Could you check a few things on this model? Use its own coordinates, in mm. Round coordinates to 2 decimals unless told otherwise and drop trailing zeros. Loops run counter-clockwise (first coordinate to the right, second up) from the corner with the lowest first, then second, coordinate; pieces in that order, holes last. Notation, with made-up numbers: (23, 65) -> (55, 65) arc R29 cw to (55, 87) -> close; hole circle Ø8 at (13, -32). An arc over 180 degrees is marked (long way). One line per item, written item: value.
```python
from build123d import *

# Parameters (mm, degrees)
EXTRUDE_1_DEPTH     = 3
SKETCH_2_R          = 1.6
SKETCH_2_R_2        = 2.85
CUT_EXTRUDE_3_DEPTH = 1.5
SKETCH_3_R          = 7.5
SKETCH_3_R_2        = 15.25
CUT_EXTRUDE_4_DEPTH = 3


with BuildPart() as part:
    # 草图1 → 凸台-拉伸1 (new body)
    with BuildSketch(Plane(origin=(0, 0, 0), x_dir=(1, 0, 0), z_dir=(0, 1, 0))):
        Polygon((5, 48), (71, 48), (71, 5), (75, 5), (75, -5), (71, -5), (71, -48), (5, -48), (5, -51), (-5, -51), (-5, -48), (-71, -48), (-71, -5), (-75, -5), (-75, 5), (-71, 5), (-71, 48), (-5, 48), (-5, 51), (5, 51), align=None)
    extrude(amount=EXTRUDE_1_DEPTH)

    # 草图2 → 切除-拉伸3 (cut)
    with BuildSketch(Plane(origin=(0, 3, 0), x_dir=(1, 0, 0), z_dir=(0, 1, 0))):
        with Locations(Location((-61, -33, 0), (0, 0, 270))):
            Circle(SKETCH_2_R)
        with Locations(Location((24, -33, 0), (0, 0, 270))):
            Circle(SKETCH_2_R)
        with Locations(Location((-61, -11, 0), (0, 0, 270))):
            Circle(SKETCH_2_R_2)
        with Locations(Location((24, -11, 0), (0, 0, 270))):
            Circle(SKETCH_2_R_2)
        with Locations(Location((-61.99896854, 10.977307885, 0), (0, 0, 270))):
            Circle(SKETCH_2_R)
        with Locations(Location((23.00103146, 10.977307885, 0), (0, 0, 270))):
            Circle(SKETCH_2_R)
    extrude(amount=-CUT_EXTRUDE_3_DEPTH, mode=Mode.SUBTRACT)

    # 草图3 → 切除-拉伸4 (cut)
    with BuildSketch(Plane(origin=(0, 3, 0), x_dir=(1, 0, 0), z_dir=(0, 1, 0))):
        with Locations(Location((-18.5, -11, 0), (0, 0, 270))):
            Circle(SKETCH_3_R)
        with Locations(Location((49, -21, 0), (0, 0, 270))):
            Circle(SKETCH_3_R_2)
        with Locations(Location((49, 21, 0), (0, 0, 270))):
            Circle(SKETCH_3_R_2)
    extrude(amount=-CUT_EXTRUDE_4_DEPTH, mode=Mode.SUBTRACT)


solid = part.part
```
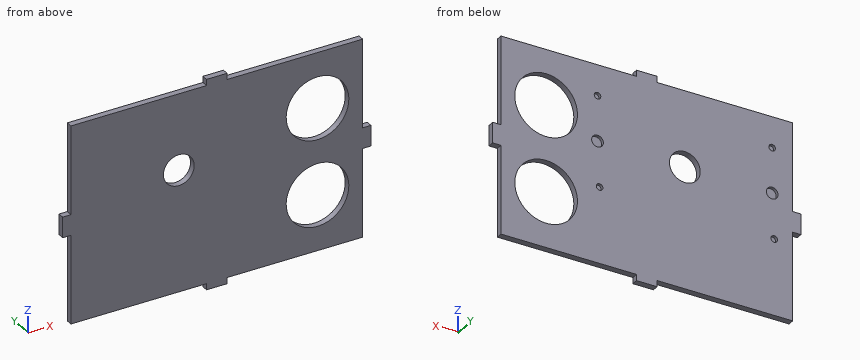
Item 1: If we section it at D-D on y = 2.45: Count the separate pieces of the cut face and the enclosed holes in it, plus the area to 3 significant figures.
Output:
separate pieces: 1
enclosed holes: 9
area: 12,100 mm²
Item 2: I need wall thicknesses on line 1 (X direction, y = 2.25, z = 21); line 2 (X direction, y = 1.6, z = 7.5); line 3 (X direction, y = 1.35, z = -7). Which ranges of each line are inside material? Lowest first, please. Write a range as from..to.
Output:
line 1: x = -71..33.75, 64.25..71
line 2: x = -71..-25.13, -11.87..41.91, 56.09..71
line 3: x = -71..42.95, 55.05..71
Item 3: If we section it at C-C on x = 56: List the corners of the cut face in (y, z) for me, plus the area to 3 significant figures.
Output:
outline: (0, -48) -> (3, -48) -> (3, -34.55) -> (0, -34.55) -> close; (0, -7.45) -> (3, -7.45) -> (3, 7.45) -> (0, 7.45) -> close; (0, 34.55) -> (3, 34.55) -> (3, 48) -> (0, 48) -> close
area: 125 mm²
Item 4: Will these pins go through, and if not, where does the flat tip stop? pin 1 Ø1.5 at (x, y) = (72.5, 1.5) entering from -Z; pin 2 Ø1.5 at (x, y) = (72.5, 1.5) entering from +Z; pin 3 Ø4.5 at (x, z) = (-61, 11) entering from +Y.
Output:
pin 1: stops at z = -5
pin 2: stops at z = 5
pin 3: stops at y = 1.5
Item 5: If we section it at B-B on z = 21: List the corners of the cut face in (x, y) for me.
Output:
outline: (-71, 0) -> (33.75, 0) -> (33.75, 3) -> (-71, 3) -> close; (64.25, 0) -> (71, 0) -> (71, 3) -> (64.25, 3) -> close
Item 6: If we section it at A-A on x = -18.5: List the corners of the cut face in (y, z) for me, plus the area to 3 significant figures.
Output:
outline: (0, -48) -> (3, -48) -> (3, 3.5) -> (0, 3.5) -> close; (0, 18.5) -> (3, 18.5) -> (3, 48) -> (0, 48) -> close
area: 243 mm²
